Input: part model. Units: mm. Frame: model coordinates. A direction names the side the tool comes from. Coordinates: 2 decimals unless noted, no trailing zeros. Write each loop counter-clockwise with the first axis right and the second up, starting at its lowest first coordinate (ties: lowest second). Pieces come first, ordered by that corner, then holes. Notation, with made-up numbers: M 47.5,15 L 56.5,15 A28 ccw 56.5,53 Z; hole C 65,-12 d11. An arc over 180 degrees is marked long. Write each question's results on one line, items separated by ' | '. Start each with the question number.
1. First-contact query: pin 1 (3 mm diameter, centred on x = 49, y = 6.5, fed in from +Z); pin 2 (3 mm diameter, centred on y = 52, z = -48, fed in from -X); pin 3 (2.5 mm diameter, centred on y = 90.5, z = 4.5, fed in from -X). Flat tips, straight axial feed; report the tip coordinate or a pass-through.
2. Set-up query: faces 1 (the flat face through (50, 15, -8)), 2 (the flat face through (22, 10, -48)), 3 (the flat face through (68, 10, 8)), 4 (the flat face through (80, 74, 4)). Return all of +Z, -Z, +X, -X, +Y, -Y with unobstructed straight access to the full face (end or side cutting, diameter ignored); none if empty.
3. Ray query, probe 1 along X at (y, z) = (14.5, 10.5); probe 2 along Z at (x, y) = (6, 36.5); probe 3 along X at (y, z) = (13.5, -40.5). Return the intervals inside material, ascending.
4. Section query C-C, the plane x = 57. Output: boundary loops of the cut face in (y, z).
5. Section query D-D, the plane y = 14. Output: boundary loops of the cut face in (x, z).
6. Pull-direction query (X, two-part tool) for faces 5 (the flat face through (-46, 15, 8)), 6 (the flat face through (-48, 10, 8)), 7 (the cylindrical face through (85, 135, 3)); classes: +X half, -X half, draft (parallel to the pull), parting line (faces both ways), or undercut.
7. Section query A-A, the plane y = 53. Output: boundary loops of the cut face in (x, z), and give its area (3 significant figures).
8. Section query B-B, the plane z = 10. Output: boundary loops of the cut face in (x, y).
```python
from build123d import *

# Parameters (mm, degrees)
EXTRUDE_1_DEPTH     = 10
EXTRUDE_2_DEPTH     = 10
SKETCH_4_W          = 32
SKETCH_4_H          = 4
EXTRUDE_3_DEPTH     = 60
CUT_EXTRUDE_1_DEPTH = 30
SKETCH_6_W          = 12
SKETCH_6_H          = 10
EXTRUDE_4_DEPTH     = 40
SKETCH_7_W          = 10
SKETCH_7_H          = 5
EXTRUDE_5_DEPTH     = 110
SKETCH_8_R          = 5
EXTRUDE_6_DEPTH     = 5


with BuildPart() as part:
    # 草图1 → 凸台-拉伸1 (new body)
    with BuildSketch(Plane(origin=(0, 0, 0), x_dir=(1, 0, 0), z_dir=(0, 1, 0))):
        with BuildLine():
            Line((-50, 0), (-46, 0))
            ThreePointArc((-46, 0), (0, 46), (46, 0))
            Line((46, 0), (50, 0))
            ThreePointArc((50, 0), (0, 50), (-50, 0))
        make_face()
    extrude(amount=EXTRUDE_1_DEPTH)

    # 草图3 → 凸台-拉伸2 (add)
    with BuildSketch(Plane(origin=(0, 10, 0), x_dir=(1, 0, 0), z_dir=(0, 1, 0))):
        with BuildLine():
            Line((-50, 16), (-47.370877129, 16))
            ThreePointArc((-47.370877129, 16), (-36.689752119, 33.968545589), (-19.595917942, 46))
            Line((-19.595917942, 46), (-30, 46))
            Line((-30, 46), (-30, 50))
            Line((-30, 50), (30, 50))
            Line((30, 50), (30, 46))
            Line((30, 46), (19.595917942, 46))
            ThreePointArc((19.595917942, 46), (36.689752119, 33.968545589), (47.370877129, 16))
            Line((47.370877129, 16), (50, 16))
            Line((50, 16), (50, -16))
            Line((50, -16), (46, -16))
            Line((46, -16), (46, 0))
            ThreePointArc((46, 0), (0, 46), (-46, 0))
            Line((-46, 0), (-46, -16))
            Line((-46, -16), (-50, -16))
            Line((-50, -16), (-50, 16))
        make_face()
    extrude(amount=EXTRUDE_2_DEPTH)

    # 草图4 → 凸台-拉伸3 (add)
    with BuildSketch(Plane(origin=(0, 20, 0), x_dir=(1, 0, 0), z_dir=(0, 1, 0))):
        with Locations((0, 48)):
            Rectangle(SKETCH_4_W, SKETCH_4_H)
    extrude(amount=EXTRUDE_3_DEPTH)

    # 草图5 → 切除-拉伸1 (cut)
    with BuildSketch(Plane(origin=(0, 0, -50), x_dir=(-1, 0, 0), z_dir=(0, 0, -1))):
        with BuildLine():
            Line((-16, 64), (-16, 97.905328476))
            Line((-16, 97.905328476), (16, 97.905328476))
            Line((16, 97.905328476), (16, 64))
            ThreePointArc((16, 64), (0, 80), (-16, 64))
        make_face()
    extrude(amount=-CUT_EXTRUDE_1_DEPTH, mode=Mode.SUBTRACT)

    # 草图6 → 凸台-拉伸4 (add)
    with BuildSketch(Plane(origin=(50, 0, 0), x_dir=(0, 0, -1), z_dir=(1, 0, 0))):
        with Locations((-7, 15)):
            Rectangle(SKETCH_6_W, SKETCH_6_H)
    extrude(amount=EXTRUDE_4_DEPTH)

    # 草图7 → 凸台-拉伸5 (add)
    with BuildSketch(Plane(origin=(0, 20, 0), x_dir=(1, 0, 0), z_dir=(0, 1, 0))):
        with Locations((85, -3.5)):
            Rectangle(SKETCH_7_W, SKETCH_7_H)
    extrude(amount=EXTRUDE_5_DEPTH)

    # 草图8 → 凸台-拉伸6 (add)
    with BuildSketch(Plane(origin=(0, 0, 1), x_dir=(-1, 0, 0), z_dir=(0, 0, -1))):
        with Locations((-85, 130)):
            Circle(SKETCH_8_R)
    extrude(amount=-EXTRUDE_6_DEPTH)


solid = part.part
```
Answer:
1) pin 1: z = 0 | pin 2: x = -16 | pin 3: x = 80
2) face 1: -Z, +X, +Y, -Y | face 2: -Z, +X, -Y | face 3: +Z, +X, -X, -Y | face 4: +Z, -Z, -X, +Y
3) probe 1: -50 to -46, 46 to 90 | probe 2: -50 to -46 | probe 3: -29.32 to -21.81, 21.81 to 29.32
4) outline: M 10,1 L 20,1 L 20,13 L 10,13 Z
5) outline: M -50,-16 L -47.37,-16 A50 ccw -19.6,-46 L -30,-46 L -30,-50 L 30,-50 L 30,-46 L 19.6,-46 A50 ccw 47.37,-16 L 50,-16 L 50,1 L 90,1 L 90,13 L 50,13 L 50,16 L 46,16 L 46,0 A46 cw -46,0 L -46,16 L -50,16 Z
6) face 5: undercut | face 6: draft | face 7: parting line
7) outline: M -16,-50 L 16,-50 L 16,-46 L -16,-46 Z; M 80,1 L 90,1 L 90,6 L 80,6 Z | area: 178 mm^2
8) outline: M -50,10 L -46,10 L -46,20 L -50,20 Z; M 46,10 L 90,10 L 90,20 L 46,20 Z
